Part model, mm, in its own coordinate system. A direction names the side the tool comes from. Round coordinates to 2 decimals unless told otherwise and drop trailing zeros. Write each loop counter-clockwise with the first axis right and the second up, starting at its lowest first coordinate (ties: lowest second). Pieces come first, ordered by that corner, then holes. Notation, with made-up numbers: M 74,85 L 102,85 A32 ccw 102,115 Z; hole C 47,23.25 d11. An arc over 180 degrees is marked long. Use a Markdown table: item, result. Add a question column.
1) Slice it at A-A on y = -32. Write the cut outline in (x, z), plus the area to 3 significant figures.
2) Slice it at D-D on y = -7.5. Write the cut outline in (x, z).
3) Two-plate mould, pull along Y, no slides. Class faces 1 (the face through (15.4, -5.1, 21)), 2 (the face through (-1.86, -31.69, 4.93)), 3 (the face through (76.049, -34.298, 5.07)): released by +Y, released by -Y, zero draft, split by the parting line, or undercut.
4) Which spindle directions (+Z, -Z, +X, -X, +Y, -Y) get a long thin tool onto all of the face, cutting with end or side? Do faces 4 (the face through (-27.494, -5, 30)), 5 (the face through (10, -22, 10)), 6 (the face through (-11.494, -5, 36)), 7 (the face through (58, -32, 10)). Say none if no direction does.
5) Wall check: probe 1 along X at (y, z) = (-9.5, 31); probe 2 along Y at (x, z) = (-9, 18); probe 3 along X at (y, z) = (-3, 50). Give the ranges that are in metal, low to high.
6) Slice it at C-C on z = 30.5. Write the cut outline in (x, y).
7) Slice it at B-B on x = 16.5. Write the cut outline in (y, z), plus the area to 3 significant figures.
8) Drop flat-ended pins along their axis: P1, Ø11, axis at y = -5.5, z = 34.5, coming from the +X side; P2, Ø22, axis at y = -37, z = 22.5, coming from the -X side; P3, Ø1, axis at x = 45.5, y = -41, coming from the +Z side. Give the stop position or say it passes through.
```python
from build123d import *

# Parameters (mm, degrees)
F0_W      = 10
F0_H      = 44
F1_DEPTH  = 60
F0_W_2    = 48
F2_DEPTH  = 10
F4_DEPTH  = 25
F6_DEPTH  = 25
F7_R      = 6
F8_DEPTH  = 10.001
F10_DEPTH = 10.001


with BuildPart() as f1:
    # F0 (on Top) → F1 (new body)
    with BuildSketch(Plane.XY):
        Polygon((82.506062, 0), (-27.493938, 0), (-27.493938, -10), (24.506062, -10), (34.506062, -10), (82.506062, -10), align=None)
        with Locations((29.506062, -32)):
            Rectangle(F0_W, F0_H)
    extrude(amount=F1_DEPTH)

    # F0 (on Top) → F2 (join)
    with BuildSketch(Plane.XY):
        Polygon((24.506062, -10), (-27.493938, -10), (24.506062, -54), align=None)
        with Locations((58.506062, -32)):
            Rectangle(F0_W_2, F0_H)
    extrude(amount=F2_DEPTH)

    # F3 (on face) → F4 (cut)
    with BuildSketch(Plane.YZ.offset(34.506062)):
        Polygon((-54, 60), (-54, 10), (-10, 60), align=None)
    extrude(amount=-F4_DEPTH, mode=Mode.SUBTRACT)

    # F5 (on face) → F6 (cut)
    with BuildSketch(Plane.XZ.offset(10)):
        Polygon((82.506062, 60), (34.506062, 60), (82.506062, 10), align=None)
    extrude(amount=-F6_DEPTH, mode=Mode.SUBTRACT)

    # F7 (on face) → F8 (cut, through all)
    with BuildSketch(Plane.XY.offset(10)):
        with Locations((48.506062, -32)):
            Circle(F7_R)
        with Locations((70.506062, -32)):
            Circle(F7_R)
    extrude(amount=-F8_DEPTH, mode=Mode.SUBTRACT)

    # F9 (on face) → F10 (cut, through all)
    with BuildSketch(Plane.XZ.offset(10)):
        with BuildLine():
            ThreePointArc((-1.493938, 46), (-6.493938, 51), (-11.493938, 46))
            Line((-11.493938, 46), (-11.493938, 26))
            ThreePointArc((-11.493938, 26), (-6.493938, 21), (-1.493938, 26))
            Line((-1.493938, 26), (-1.493938, 46))
        make_face()
        with BuildLine():
            ThreePointArc((20.506062, 46), (15.506062, 51), (10.506062, 46))
            Line((10.506062, 46), (10.506062, 26))
            ThreePointArc((10.506062, 26), (15.506062, 21), (20.506062, 26))
            Line((20.506062, 26), (20.506062, 46))
        make_face()
    extrude(amount=-F10_DEPTH, mode=Mode.SUBTRACT)


solid = f1.part
```
Entries:
| question | item | result |
|---|---|---|
| 1 | outline | M -1.49,0 L 42.51,0 L 42.51,10 L 34.51,10 L 34.51,35 L 24.51,35 L 24.51,10 L -1.49,10 Z; M 54.51,0 L 64.51,0 L 64.51,10 L 54.51,10 Z; M 76.51,0 L 82.51,0 L 82.51,10 L 76.51,10 Z |
| 1 | area | 850 mm^2 |
| 2 | outline | M -27.49,0 L 82.51,0 L 82.51,10 L 34.51,60 L -27.49,60 Z; hole M -11.49,26 A5 ccw -1.49,26 L -1.49,46 A5 ccw -11.49,46 Z; hole M 10.51,26 A5 ccw 20.51,26 L 20.51,46 A5 ccw 10.51,46 Z |
| 3 | face 1 | zero draft |
| 3 | face 2 | released by -Y |
| 3 | face 3 | undercut |
| 4 | face 4 | +Z, -Z, -X, +Y, -Y |
| 4 | face 5 | +Z, -X, -Y |
| 4 | face 6 | +Y, -Y |
| 4 | face 7 | +Z, +X, -Y |
| 5 | probe 1 | x = -27.49 to -11.49, -1.49 to 10.51, 20.51 to 62.35 |
| 5 | probe 2 | y = -10 to 0 |
| 5 | probe 3 | x = -27.49 to -9.49, -3.49 to 12.51, 18.51 to 44.11 |
| 6 | outline | M -27.49,-10 L -11.49,-10 L -11.49,0 L -27.49,0 Z; M -1.49,-10 L 10.51,-10 L 10.51,0 L -1.49,0 Z; M 20.51,-10 L 24.51,-10 L 24.51,-35.96 L 34.51,-35.96 L 34.51,-10 L 62.83,-10 L 62.83,0 L 20.51,0 Z |
| 7 | outline | M -47.23,0 L 0,0 L 0,21.1 L -10,21.1 L -10,10 L -47.23,10 Z; M -10,50.9 L 0,50.9 L 0,60 L -10,60 Z |
| 7 | area | 674 mm^2 |
| 8 | P1 | stops at x = 64.27 |
| 8 | P2 | stops at x = 24.51 |
| 8 | P3 | stops at z = 10 |
